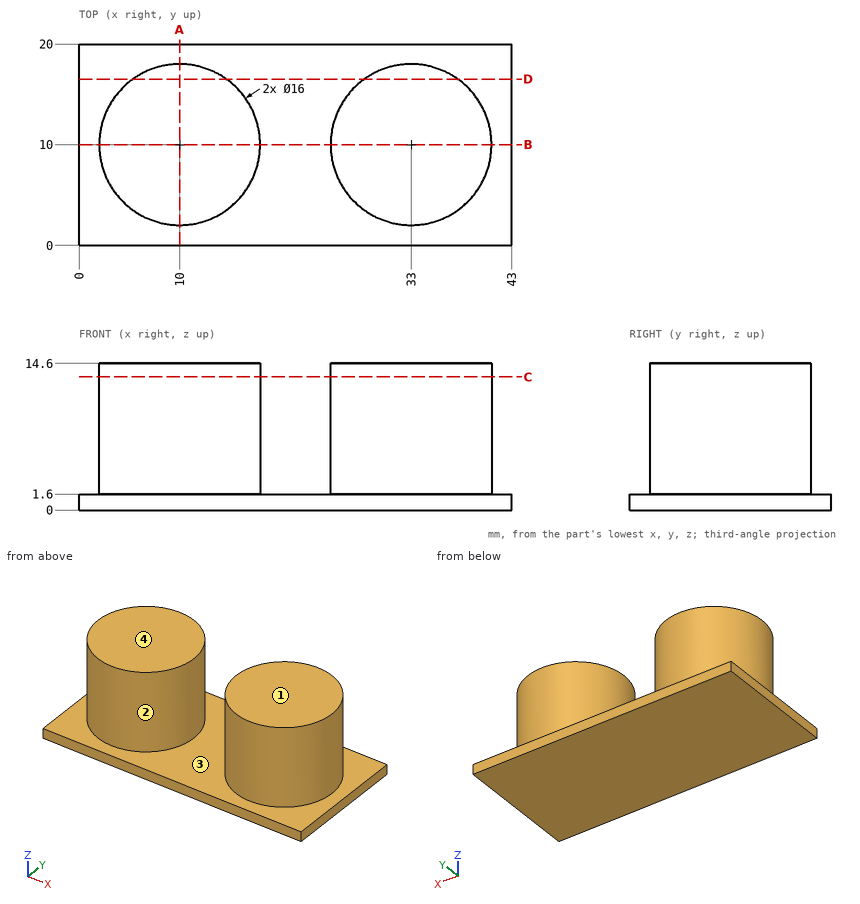
Input: dimensioned drawing with shaded views. Units: mm. Origin: part minimum x, y, z. A direction names the side the tool comes from. Round coordinates to 2 decimals unless told otherwise and drop trailing zeros. Order: outer loops, then holes, each group sorted by start corner. A loop starts at its lowest first (then second) coordinate and runs counter-clockwise, first axis right, second up. Notation, with made-up numbers: (-12, 73.5) - (28, 73.5) arc R32 cw to (28, 106.5) - close; hole circle Ø7 at (-21, 57). An arc over 180 degrees is marked (long way). Use CSV: the item, a comma, the result in double quotes. Start each with the question number.
Q1. Access query for the marked faces 3 and 4. Directions: +Z, -Z, +X, -X, +Y, -Y. A direction counts if a zero-diameter tool reaches every point of the face in a straight line with its end or side. Return the directions, or none.
Q2. Material intervals for line 1 along X through (y, z) = (10.25, 2); line 2 along Z through (x, y) = (6, 2.75); line 3 along X through (y, z) = (11.75, 11), sorted ascending. Write a range as from..to.
Q3. Section query A-A (x = 10). Return loops of the section in (y, z).
Q4. Section query D-D (y = 16.5). Return loops of the section in (x, z), and give its area (3 significant figures).
Q5. First-contact query: pin 1 (2 mm diameter, centred on x = 4.5, y = 2.5, fed in from -Z); pin 2 (4 mm diameter, centred on x = 22.5, z = 6, fed in from -Y). Flat tips, straight axial feed; report the tip coordinate or a pass-through.
Q6. Section query B-B (y = 10). Return loops of the section in (x, z), and give its area (3 significant figures).
Q7. Mould query, pull axis X, two halves, no side actions, for the marked faces 1 and 2. Classes: +X half, -X half, draft (parallel to the pull), parting line (faces both ways), or undercut.
Q8. Section query C-C (z = 13.25). Return loops of the section in (x, y).
Result set:
1,face 3,"+Z"
1,face 4,"+Z, +X, -X, +Y, -Y"
2,line 1,"x = 2..18, 25..41"
2,line 2,"z = 0..1.6"
2,line 3,"x = 2.19..17.81, 25.19..40.81"
3,outline,"(0, 0) - (20, 0) - (20, 1.6) - (18, 1.6) - (18, 14.6) - (2, 14.6) - (2, 1.6) - (0, 1.6) - close"
4,outline,"(0, 0) - (43, 0) - (43, 1.6) - (37.66, 1.6) - (37.66, 14.6) - (28.34, 14.6) - (28.34, 1.6) - (14.66, 1.6) - (14.66, 14.6) - (5.34, 14.6) - (5.34, 1.6) - (0, 1.6) - close"
4,area,"311 mm2"
5,pin 1,"stops at z = 0"
5,pin 2,"passes through"
6,outline,"(0, 0) - (43, 0) - (43, 1.6) - (41, 1.6) - (41, 14.6) - (25, 14.6) - (25, 1.6) - (18, 1.6) - (18, 14.6) - (2, 14.6) - (2, 1.6) - (0, 1.6) - close"
6,area,"485 mm2"
7,face 1,"draft"
7,face 2,"undercut"
8,outline,"circle Ø16 at (10, 10); circle Ø16 at (33, 10)"
